The figure shows three views and two pictorial views of one solid part (mm, origin at its lowest corner). Answer the questions. A direction names the side the tool comes from. Coordinates: 2 decimals unless noted, no trailing zeros. Order: outer loops, then holes, each group sorted by start corner. A loop starts at its lowest first (then second) coordinate and runs counter-clockwise, first axis right, second up. Notation, with made-up numbers: (47.5, 68.5) -> (63.5, 68.5) arc R20 cw to (63.5, 87.5) -> close; hole circle Ø11 at (25, 78). An arc over 180 degrees is marked (long way). Return JSON: item names as keys, results as strings.
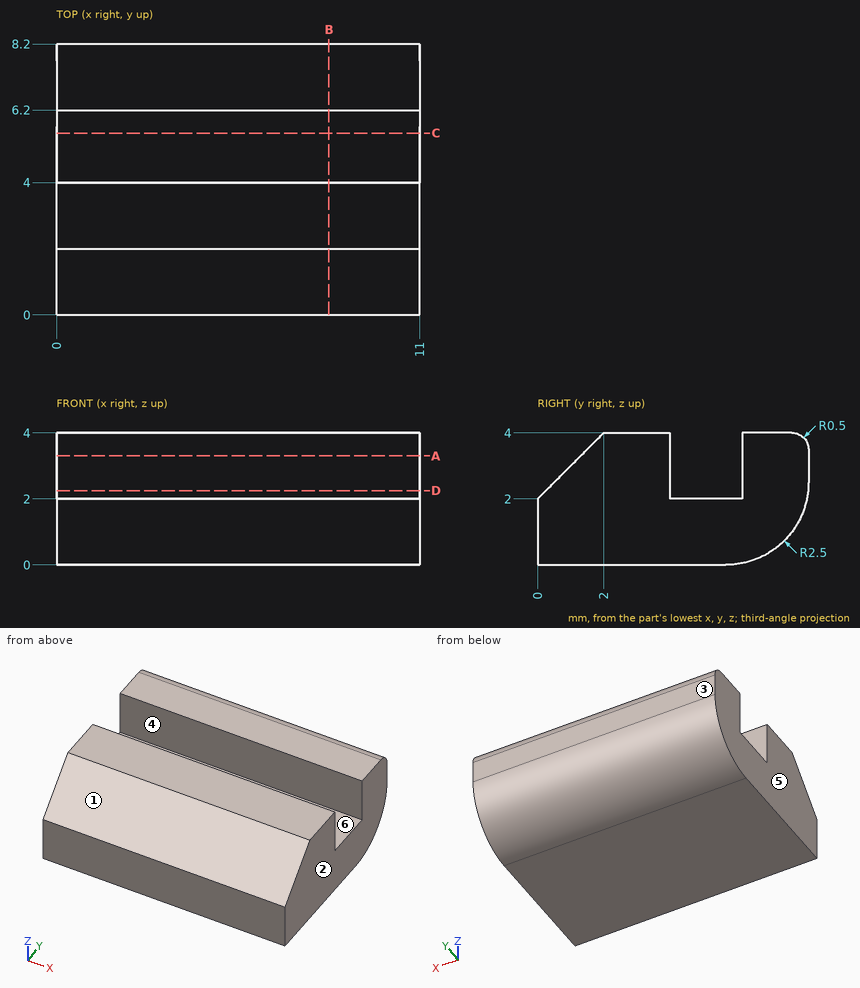
1. The part is cut by section A-A on z = 3.3. Give the vertices of the cut face in (x, y), and give its area (3 significant figures).
Answer block:
{"outline": "(0, 1.3) -> (11, 1.3) -> (11, 4) -> (0, 4) -> close; (0, 6.2) -> (11, 6.2) -> (11, 8.2) -> (0, 8.2) -> close", "area": "51.7 mm2"}
2. The part is cut by section B-B on x = 8.25. Give the vertices of the cut face in (y, z).
Answer block:
{"outline": "(0, 0) -> (5.7, 0) arc R2.5 ccw to (8.2, 2.5) -> (8.2, 3.5) arc R0.5 ccw to (7.7, 4) -> (6.2, 4) -> (6.2, 2) -> (4, 2) -> (4, 4) -> (2, 4) -> (0, 2) -> close"}
3. The part is cut by section D-D on z = 2.25. Give the vertices of the cut face in (x, y), and give its area (3 significant figures).
Answer block:
{"outline": "(0, 0.25) -> (11, 0.25) -> (11, 4) -> (0, 4) -> close; (0, 6.2) -> (11, 6.2) -> (11, 8.19) -> (0, 8.19) -> close", "area": "63.1 mm2"}
4. Consider line 1 (Y direction, x = 5.5, z = 3.6); line 2 (Y direction, x = 1.25, z = 3.65); line 3 (Z direction, x = 8, y = 1.5). Determine where each line is inside the solid, lowest interval first. Write a range as from..to.
Answer block:
{"line 1": "y = 1.6..4, 6.2..8.19", "line 2": "y = 1.65..4, 6.2..8.18", "line 3": "z = 0..3.5"}
5. Determine the mould class of the marked faces 1, 2, 3 and 4 for opening direction Y: pulls with the +Y half, pulls with the -Y half, needs draft (parallel to the pull), parting line crosses it, or undercut.
Answer block:
{"face 1": "pulls with the -Y half", "face 2": "needs draft", "face 3": "pulls with the +Y half", "face 4": "undercut"}
6. The part is cut by section C-C on y = 5.5. Give the vertices of the cut face in (x, z).
Answer block:
{"outline": "(0, 0) -> (11, 0) -> (11, 2) -> (0, 2) -> close"}
7. This flat-tipped pin is pushed along its axis until it touches: pin 1 Ø1.8 at (x, y) = (3, 5) entering from +Z. Where does it stop, or does it pass through?
Answer block:
{"pin 1": "stops at z = 2"}
8. For the marked faces 5 and 6, determine the directions among +Z, -Z, +X, -X, +Y, -Y from which every point of the face is accessible in a straight line to the end or side of a thin tool.
Answer block:
{"face 5": "+Z, -Z, -X, +Y, -Y", "face 6": "+Z, +X, -X"}
